Build history of the part. All positions in model axes, mm. A direction names the side the tool comes from. Round coordinates to 2 decimals unless told otherwise and drop trailing zeros. Write each loop counter-clockwise with the first axis right and the second up, starting at its lowest first coordinate (ties: lowest second). Pieces come first, ordered by that corner, then holes. Notation, with made-up numbers: (4, -12.5) -> (31, -12.5) arc R15 cw to (31, 15.5) -> close; hole circle Ø1 at (62, 86.25). An arc over 180 degrees is marked (long way). Answer in a Markdown table with one row per item.
```python
from build123d import *

# Parameters (mm, degrees)
SKETCH1_W                 = 66
SKETCH1_H                 = 28.2
BOSS_EXTRUDE1_DEPTH       = 3
BOSS_EXTRUDE4_DEPTH       = 7
SKETCH17_R                = 1.75
BOSS_EXTRUDE7_DEPTH       = 0.75
REVOLVE4_ANGLE            = 180
LPATTERN2_COUNT           = 2
LPATTERN2_PITCH           = 30
LPATTERN2_COPY_1_DEPTH    = 7
LPATTERN2_COPY_2_SKETCH_R = 1.75
LPATTERN2_COPY_2_DEPTH    = 0.75
LPATTERN2_COPY_3_ANGLE    = 180
FILLET5_R                 = 1.5
BOSS_EXTRUDE3_DEPTH       = 3


with BuildPart() as part:
    # Sketch1 → Boss-Extrude1 (new body)
    with BuildSketch(Plane.XY):
        Rectangle(SKETCH1_W, SKETCH1_H)
    extrude(amount=BOSS_EXTRUDE1_DEPTH)

    # Sketch10 → Boss-Extrude4 (add)
    with BuildSketch(Plane.ZY.offset(33)):
        with BuildLine():
            Line((0, 19.1), (0, 14.1))
            Line((0, 14.1), (3, 14.1))
            Line((3, 14.1), (3, 16.1))
            ThreePointArc((3, 16.1), (5.121320344, 21.221320344), (0, 19.1))
        make_face()
    boss_extrude4 = extrude(amount=-BOSS_EXTRUDE4_DEPTH)

    # Sketch17 → Boss-Extrude7 (add)
    with BuildSketch(Plane(origin=(-26, 0, 0), x_dir=(0, 0, -1), z_dir=(1, 0, 0))):
        with Locations(Location((-3, 19.1, 0), (0, 0, 180))):
            Circle(SKETCH17_R)
    boss_extrude7 = extrude(amount=BOSS_EXTRUDE7_DEPTH)

    # Sketch18 → Revolve4 (revolve)
    with BuildSketch(Plane(origin=(-25.25, 0, 0), x_dir=(0, 0, -1), z_dir=(1, 0, 0))):
        with BuildLine():
            Line((-3, 20.85), (-3, 17.35))
            ThreePointArc((-3, 17.35), (-1.25, 19.1), (-3, 20.85))
        make_face()
    revolve4 = revolve(axis=Axis((-25.25, 20.85, 3), (0, -1, 0)), revolution_arc=REVOLVE4_ANGLE)

    # Mirror1: Boss-Extrude4, Boss-Extrude7, Revolve4 across plane
    add(boss_extrude4.mirror(Plane(origin=(-21.625, 0, 0), x_dir=(0, 0, 1), z_dir=(1, 0, 0))))
    add(boss_extrude7.mirror(Plane(origin=(-21.625, 0, 0), x_dir=(0, 0, 1), z_dir=(1, 0, 0))))
    add(revolve4.mirror(Plane(origin=(-21.625, 0, 0), x_dir=(0, 0, 1), z_dir=(1, 0, 0))))

    # LPattern2: Boss-Extrude4, Boss-Extrude7, Revolve4 ×2
    with Locations(*[(i * LPATTERN2_PITCH, 0, 0) for i in range(1, LPATTERN2_COUNT)]):
        add(boss_extrude4)
        add(boss_extrude7)
        add(revolve4)

    # LPattern2 copy 1 sketch → LPattern2 copy 1 (add)
    with BuildSketch(Plane(origin=(19.75, 0, 0), x_dir=(0, 0, 1), z_dir=(1, 0, 0))):
        with BuildLine():
            Line((0, -19.1), (0, -14.1))
            Line((0, -14.1), (3, -14.1))
            Line((3, -14.1), (3, -16.1))
            ThreePointArc((3, -16.1), (5.121320344, -21.221320344), (0, -19.1))
        make_face()
    extrude(amount=-LPATTERN2_COPY_1_DEPTH)

    # LPattern2 copy 2 sketch → LPattern2 copy 2 (add)
    with BuildSketch(Plane(origin=(12.75, 0, 0), x_dir=(0, 0, -1), z_dir=(-1, 0, 0))):
        with Locations((-3, -19.1)):
            Circle(LPATTERN2_COPY_2_SKETCH_R)
    extrude(amount=LPATTERN2_COPY_2_DEPTH)

    # LPattern2 copy 3 sketch → LPattern2 copy 3 (revolve)
    with BuildSketch(Plane(origin=(12, 0, 0), x_dir=(0, 0, -1), z_dir=(-1, 0, 0))):
        with BuildLine():
            Line((-3, -20.85), (-3, -17.35))
            ThreePointArc((-3, -17.35), (-1.25, -19.1), (-3, -20.85))
        make_face()
    revolve(axis=Axis((12, 20.85, 3), (0, 1, 0)), revolution_arc=LPATTERN2_COPY_3_ANGLE)

    # Fillet5
    fillet5_edges = [part.edges().sort_by_distance(p)[0] for p in [
        (-33, 21.221320344, 5.121320344),
        (0, -14.1, 0),
        (-33, 2.5, 0),
        (33, 0, 0),
    ]]
    fillet(fillet5_edges, radius=FILLET5_R)

    # Sketch9 → Boss-Extrude3 (add)
    with BuildSketch(Plane.XY.offset(3)):
        Polygon((-31.7, 11.6), (-30.7, 11.6), (-30.7, -11.85), (30.7, -11.85), (30.7, 11.6), (31.7, 11.6), (31.7, -11.85), (31.7, -12.85), (-30.7, -12.85), (-31.7, -12.85), align=None)
    extrude(amount=BOSS_EXTRUDE3_DEPTH)


solid = part.part
```
Q1. Drop flat-ended pins along their axis: P1, Ø3.5, axis at y = 3, z = 5, coming from the +X side; P2, Ø6, axis at x = 8.5, y = 13, coming from the +Z side; P3, Ø0.9, axis at y = -1, z = 4.5, coming from the -X side. Give the stop position or say it passes through.
A:
| item | result |
|---|---|
| P1 | x = 31.7 |
| P2 | z = 3 |
| P3 | x = -31.7 |
Q2. Saw through at A-A on x = 3. Write the cut outline in (y, z), plus the area to 3 significant figures.
A:
| item | result |
|---|---|
| outline | (-14.1, 1.5) arc R1.5 ccw to (-12.6, 0) -> (19.1, 0) arc R3 ccw (long way) to (16.1, 3) -> (-11.85, 3) -> (-11.85, 6) -> (-12.85, 6) -> (-12.85, 3) -> (-14.1, 3) -> close |
| area | 123 mm² |
Q3. Saw through at B-B on y = -3. Write the cut outline in (x, z), plus the area to 3 significant figures.
A:
| item | result |
|---|---|
| outline | (-33, 1.5) arc R1.5 ccw to (-31.5, 0) -> (31.5, 0) arc R1.5 ccw to (33, 1.5) -> (33, 3) -> (31.7, 3) -> (31.7, 6) -> (30.7, 6) -> (30.7, 3) -> (-30.7, 3) -> (-30.7, 6) -> (-31.7, 6) -> (-31.7, 3) -> (-33, 3) -> close |
| area | 203 mm² |
Q4. Which spindle directions (+Z, -Z, +X, -X, +Y, -Y) get a long thin tool onto all of the face, cutting with end or side? Do faces 1 (the flat face through (-22, 14.1, 1)), 2 (the flat face through (-26, 17, 2)), 3 (the flat face through (-10.25, 18, 2)), 4 (the flat face through (31.7, -1, 4)). Say none if no direction does.
A:
| item | result |
|---|---|
| face 1 | +Z, -Z |
| face 2 | none |
| face 3 | +Z, -Z, +Y |
| face 4 | +Z, +X, +Y, -Y |
Q5. Wall check: line 1 (X direction, y = 15.5, z = 1.75); line 2 (X direction, y = 5.5, z = 3.75); line 3 (Z direction, x = -30, y = 8.5). Give the ranges that are in metal, low to high. Write a range as [from, to].
A:
| item | result |
|---|---|
| line 1 | [-33, -26], [-17.25, -10.25], [-3, 4], [12.75, 19.75] |
| line 2 | [-31.7, -30.7], [30.7, 31.7] |
| line 3 | [0, 3] |
Q6. Two-plate mould, pull along X, no slides. Class faces 5 (the flat face through (0, 2, 3)), 6 (the cylindrical face through (0.46, -13.65, 0.43)), 7 (the flat face through (19.75, 18, 2)): released by +X, released by -X, zero draft, split by the parting line, or undercut.
A:
| item | result |
|---|---|
| face 5 | undercut |
| face 6 | zero draft |
| face 7 | released by +X |
